Geometry check sheet. Reference: the model listing, model coordinates, mm. A direction names the side the tool comes from. Give positions to 0.01 mm unless a question says otherwise; leave off trailing zeros. Loops run counter-clockwise (first coordinate to the right, second up) from the corner with the lowest first, then second, coordinate; pieces in that order, holes last.
1. Cross-section at B-B, the plane z = -29. Record the cut outline in (x, y), plus the area to 3 significant figures.
2. Cross-section at A-A, the plane y = -74.25. Record the cut outline in (x, z), plus the area to 3 significant figures.
3. Go/stop test with flat-tipped pins: pin 1 Ø6 at (y, z) = (-78, -40) entering from +X; pin 2 Ø1.9 at (x, y) = (191, -83.5) entering from -Z; pin 3 Ø5 at (x, y) = (206, -84.5) entering from +Z; pin 4 Ø5 at (y, z) = (-79.5, -17) entering from +X. Record where each tip stops, or that it passes through.
4. Release check for a two-part mould opening along Z. For faces 1 (the flat face through (191, -85, -45)), 2 (the flat face through (218, -73, 0)), 3 (the flat face through (215.24, -74.21, 3.04)) record: +Z half, -Z half, draft (parallel to the pull), parting line (faces both ways), or undercut.
5. Cross-section at C-C, the plane x = 210. Record the cut outline in (y, z), plus the area to 3 significant figures.
6. Cross-section at D-D, the plane z = 2.5. Record the cut outline in (x, y).
7. Tool access check on faces 4 (the flat face through (215.24, -74.21, -46.48)), 5 (the flat face through (193.234, -83.59, -46.479)), 6 (the flat face through (193.234, -83.59, 3.042)), 7 (the flat face through (219.837, -72.245, -22.185)). Record the directions out of +Z, -Z, +X, -X, +Y, -Y that give a thin tool (end or side, any length) a straight path to the whole face; none if there is none.
8. Material ranges on L1, parallel to Y at x = 206.5, z = -33.5; L2, parallel to X at y = -77, z = 3; L3, parallel to X at y = -84, z = -4.5, recorded low to high.
from build123d import *

# Parameters (mm, degrees)
ESTRUSIONE_ESTRUSIONE1_DEPTH      = 48
ESTRUSIONE_ESTRUSIONE1_DEPTH_BACK = 6
SCHIZZO2_W                        = 45
SCHIZZO2_H                        = 2
ESTRUSIONE_ESTRUSIONE2_DEPTH      = 5
CORPO_SPOSTA_COPIA1_START         = 139.953637561
CORPO_SPOSTA_COPIA1_OUTLINE_W     = 2
CORPO_SPOSTA_COPIA1_OUTLINE_H     = 42
CORPO_SPOSTA_COPIA1_DEPTH         = 33.920640211
CORPO_SPOSTA_COPIA1_2_OUTLINE_W   = 2
CORPO_SPOSTA_COPIA1_2_OUTLINE_H   = 6
CORPO_SPOSTA_COPIA1_2_DEPTH       = 5
CORPO_SPOSTA_COPIA1_START_2       = 168.874277772
CORPO_SPOSTA_COPIA1_3_OUTLINE_W   = 2
CORPO_SPOSTA_COPIA1_3_OUTLINE_H   = 6
CORPO_SPOSTA_COPIA1_3_DEPTH       = 5
CORPO_SPOSTA_COPIA1_4_OUTLINE_W   = 2
CORPO_SPOSTA_COPIA1_4_OUTLINE_H   = 45
CORPO_SPOSTA_COPIA1_4_DEPTH       = 33.920640211
CORPO_SPOSTA_COPIA1_START_3       = 144.953637561
CORPO_SPOSTA_COPIA1_5_OUTLINE_W   = 2
CORPO_SPOSTA_COPIA1_5_OUTLINE_H   = 3
CORPO_SPOSTA_COPIA1_5_DEPTH       = 23.920640211


# Read off the part's stored shape, not the designer's step: Corpo-Sposta/copia1
with BuildPart() as part:
    # Schizzo1 → Estrusione-Estrusione1 (new, two sides: drawn at the far end of the back side and taken through both)
    with BuildSketch(Plane.XY.offset(-ESTRUSIONE_ESTRUSIONE1_DEPTH_BACK)):
        Polygon((214.839776844, -73.273463404), (192.836567017, -82.657267824), (193.62114505, -84.496951848), (215.624354877, -75.113147429), align=None)
    extrude(amount=ESTRUSIONE_ESTRUSIONE1_DEPTH + ESTRUSIONE_ESTRUSIONE1_DEPTH_BACK)

    # Schizzo2 → Estrusione-Estrusione2 (add)
    with BuildSketch(Plane(origin=(155.337655494, 66.24752432, 0), x_dir=(0, 0, -1), z_dir=(0.919842012316021, 0.39228901638767966, 0))):
        with Locations((-22.5, -152.679294766)):
            Rectangle(SCHIZZO2_W, SCHIZZO2_H)
    estrusione_estrusione2 = extrude(amount=ESTRUSIONE_ESTRUSIONE2_DEPTH)

    # Specchia1: Estrusione-Estrusione2 across plane
    add(estrusione_estrusione2.mirror(Plane(origin=(144.33605058, 61.55562211, 0), x_dir=(0, 0, 1), z_dir=(0.9198420123160211, 0.3922890163876793, 0))))

    # Corpo-Sposta/copia1 outline → Corpo-Sposta/copia1 (cut)
    with BuildSketch(Plane(origin=(0, 0, 0), x_dir=(-0.39228901638766717, 0.9198420123160262, 0), z_dir=(0.9198420123160264, 0.3922890163876671, 0)).offset(CORPO_SPOSTA_COPIA1_START)):
        with Locations((-152.679294766, 27)):
            Rectangle(CORPO_SPOSTA_COPIA1_OUTLINE_W, CORPO_SPOSTA_COPIA1_OUTLINE_H)
    extrude(amount=CORPO_SPOSTA_COPIA1_DEPTH, mode=Mode.SUBTRACT)

    # Corpo-Sposta_copia1 2 outline → Corpo-Sposta_copia1 2 (cut)
    with BuildSketch(Plane(origin=(0, 0, 0), x_dir=(-0.39228901638766717, 0.9198420123160262, 0), z_dir=(0.9198420123160264, 0.3922890163876671, 0)).offset(CORPO_SPOSTA_COPIA1_START)):
        with Locations((-152.679294766, 3)):
            Rectangle(CORPO_SPOSTA_COPIA1_2_OUTLINE_W, CORPO_SPOSTA_COPIA1_2_OUTLINE_H)
    extrude(amount=CORPO_SPOSTA_COPIA1_2_DEPTH, mode=Mode.SUBTRACT)

    # Corpo-Sposta_copia1 3 outline → Corpo-Sposta_copia1 3 (cut)
    with BuildSketch(Plane(origin=(0, 0, 0), x_dir=(-0.39228901638766717, 0.9198420123160262, 0), z_dir=(0.9198420123160264, 0.3922890163876671, 0)).offset(CORPO_SPOSTA_COPIA1_START_2)):
        with Locations((-152.679294766, 3)):
            Rectangle(CORPO_SPOSTA_COPIA1_3_OUTLINE_W, CORPO_SPOSTA_COPIA1_3_OUTLINE_H)
    extrude(amount=CORPO_SPOSTA_COPIA1_3_DEPTH, mode=Mode.SUBTRACT)

    # Corpo-Sposta_copia1 4 outline → Corpo-Sposta_copia1 4 (add)
    with BuildSketch(Plane(origin=(0, 0, 0), x_dir=(-0.39228901638766717, 0.9198420123160262, 0), z_dir=(0.9198420123160264, 0.3922890163876671, 0)).offset(CORPO_SPOSTA_COPIA1_START)):
        with Locations((-152.679294766, -22.5)):
            Rectangle(CORPO_SPOSTA_COPIA1_4_OUTLINE_W, CORPO_SPOSTA_COPIA1_4_OUTLINE_H)
    extrude(amount=CORPO_SPOSTA_COPIA1_4_DEPTH)

    # Corpo-Sposta_copia1 5 outline → Corpo-Sposta_copia1 5 (add)
    with BuildSketch(Plane(origin=(0, 0, 0), x_dir=(-0.39228901638766717, 0.9198420123160262, 0), z_dir=(0.9198420123160264, 0.3922890163876671, 0)).offset(CORPO_SPOSTA_COPIA1_START_3)):
        with Locations((-152.679294766, -46.5)):
            Rectangle(CORPO_SPOSTA_COPIA1_5_OUTLINE_W, CORPO_SPOSTA_COPIA1_5_OUTLINE_H)
    extrude(amount=CORPO_SPOSTA_COPIA1_5_DEPTH)


solid = part.part
Result:
1. outline: (188.24, -84.62) - (189.02, -86.46) - (220.22, -73.15) - (219.44, -71.31) - close
1. area: 67.8 mm2
2. outline: (212.55, -48) - (215.26, -48) - (215.26, -45) - (217.65, -45) - (217.65, 0) - (215.26, 0) - (215.26, 6) - (212.55, 6) - close
2. area: 254 mm2
3. pin 1: stops at x = 215.89
3. pin 2: stops at z = -45
3. pin 3: passes through
3. pin 4: stops at x = 211.2
4. face 1: -Z half
4. face 2: +Z half
4. face 3: draft
5. outline: (-77.51, -48) - (-75.34, -48) - (-75.34, 6) - (-77.51, 6) - close
5. area: 117 mm2
6. outline: (192.84, -82.66) - (193.62, -84.5) - (215.62, -75.11) - (214.84, -73.27) - close
7. face 4: -Z, +X, +Y
7. face 5: -Z, -X, -Y
7. face 6: +Z, -X, -Y
7. face 7: +Z, -Z, +X, +Y
8. L1: y = -79 to -76.83
8. L2: x = 206.1 to 211.2
8. L3: x = 189.69 to 194.79
